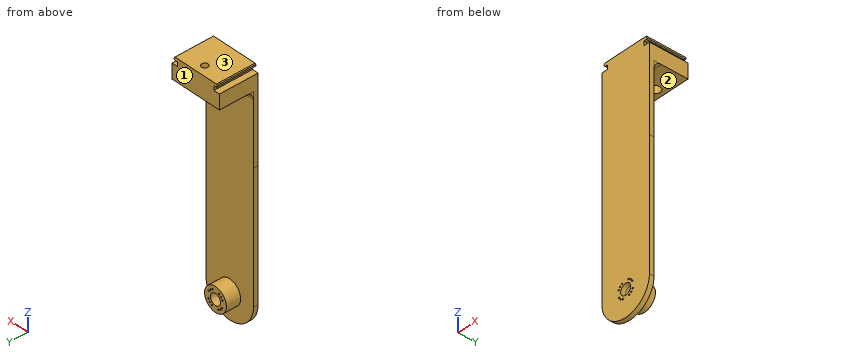
Autodesk Inventor part; units mm, degrees
ref_plane "YZ Plane" through (0, 0, 0) normal (1, 0, 0) x (0, 1, 0)
ref_plane "XZ Plane" through (0, 0, 0) normal (0, 1, 0) x (-1, 0, 0)
ref_plane "XY Plane" through (0, 0, 0) normal (0, 0, 1) x (1, 0, 0)
sketch "Sketch1" plane through (0, 0, 0) normal (0, 1, 0) x (-1, 0, 0)
  circle A0 centre (14, -52) radius 5.5 construction
  circle A1 centre (-14, -52) radius 5.5 construction
  circle A2 centre (-4.2824, 7.9159) radius 0.75 construction
  circle A3 centre (3.4651, 8.3062) radius 0.75 construction
  circle A4 centre (6.0357, 6.6761) radius 0.75 construction
  circle A5 centre (7.9159, 4.2824) radius 0.75 construction
  circle A6 centre (8.3062, -3.4651) radius 0.75 construction
  circle A7 centre (6.6761, -6.0357) radius 0.75 construction
  circle A8 centre (4.2824, -7.9159) radius 0.75 construction
  circle A9 centre (-3.4651, -8.3062) radius 0.75 construction
  circle A10 centre (-6.0357, -6.6761) radius 0.75 construction
  circle A11 centre (-7.9159, -4.2824) radius 0.75 construction
  circle A12 centre (-6.6761, 6.0357) radius 0.75 construction
  circle A13 centre (-8.3062, 3.4651) radius 0.75 construction
  circle A14 centre (0, 0) radius 6 construction
  line L0 (28, -68) -> (28, 0) construction
  arc A15 (28, 0) -> (-28, 0) centre (0, 0) ccw construction
  line L1 (-28, 0) -> (-28, -68) construction
  line L2 (-28, -68) -> (-22, -68) construction
  line L3 (-22, -68) -> (-22, -64) construction
  line L4 (-22, -64) -> (-24.8396, -64) construction
  line L5 (-24.8396, -64) -> (-25.8396, -63) construction
  line L6 (-25.8396, -63) -> (-25.8396, -61) construction
  line L7 (-25.8396, -61) -> (-24.8396, -60) construction
  line L8 (-24.8396, -60) -> (24.8396, -60) construction
  line L9 (24.8396, -60) -> (25.8396, -61) construction
  line L10 (25.8396, -61) -> (25.8396, -63) construction
  line L11 (25.8396, -63) -> (24.8396, -64) construction
  line L12 (24.8396, -64) -> (22, -64) construction
  line L13 (22, -64) -> (22, -68) construction
  line L14 (22, -68) -> (28, -68) construction
  line L15 (0, 0) -> (0, -300) construction
  line L16 (-28.3, 0) -> (-28.3, -300) construction
  line L17 (28.3, -300) -> (28.3, 0) construction
  arc A16 (28.3, 0) -> (-28.3, 0) centre (0, 0) ccw construction
  arc A17 (-28.3, -300) -> (28.3, -300) centre (0, -300) ccw construction
  line L18 (21.7, -63.7) -> (24.7153, -63.7)
  line L19 (24.7153, -63.7) -> (25.5396, -62.8757)
  line L20 (25.5396, -62.8757) -> (25.5396, -61.1243)
  line L21 (25.5396, -61.1243) -> (24.7153, -60.3)
  line L22 (24.7153, -60.3) -> (-24.7153, -60.3)
  line L23 (-24.7153, -60.3) -> (-25.5396, -61.1243)
  line L24 (-25.5396, -61.1243) -> (-25.5396, -62.8757)
  line L25 (-25.5396, -62.8757) -> (-24.7153, -63.7)
  line L26 (-24.7153, -63.7) -> (-21.7, -63.7)
  line L27 (-21.7, -63.7) -> (-21.7, -68.3)
  line L28 (-21.7, -68.3) -> (-28.3, -68.3) construction
  line L29 (-28.3, -68.3) -> (-28.3, 0) construction
  arc A18 (28.3, 0) -> (-28.3, 0) centre (0, 0) ccw construction
  line L30 (28.3, 0) -> (28.3, -68.3) construction
  line L31 (28.3, -68.3) -> (21.7, -68.3) construction
  line L32 (21.7, -68.3) -> (21.7, -63.7)
  arc A19 (-28.3, -300) -> (28.3, -300) centre (0, -300) ccw
  line L33 (0, -150) -> (28.3, -150) construction
  circle A20 centre (-4.2824, -307.9159) radius 0.75
  circle A21 centre (3.4651, -308.3062) radius 0.75
  circle A22 centre (6.0357, -306.6761) radius 0.75
  circle A23 centre (7.9159, -304.2824) radius 0.75
  circle A24 centre (8.3062, -296.5349) radius 0.75
  circle A25 centre (6.6761, -293.9643) radius 0.75
  circle A26 centre (4.2824, -292.0841) radius 0.75
  circle A27 centre (-3.4651, -291.6938) radius 0.75
  circle A28 centre (-6.0357, -293.3239) radius 0.75
  circle A29 centre (-7.9159, -295.7176) radius 0.75
  circle A30 centre (-6.6761, -306.0357) radius 0.75
  circle A31 centre (-8.3062, -303.4651) radius 0.75
  circle A32 centre (0, -300) radius 6
  line L34 (-28.3, -300) -> (-28.3, -68.3)
  line L35 (-28.3, -68.3) -> (-21.7, -68.3)
  line L36 (21.7, -68.3) -> (28.3, -68.3)
  line L37 (28.3, -68.3) -> (28.3, -300)
  point P0 (0, -150)
  dimension "d1" = 0.3
extrude "Extrusion1" add sketch "Sketch1" against normal blind 5
sketch "Sketch2" plane through (0, 0, 0) normal (0, 1, 0) x (1, 0, 0)
  circle A0 centre (0, 300) radius 6 construction
  circle A1 centre (8.3062, 303.4651) radius 0.75 construction
  circle A2 centre (6.6761, 306.0357) radius 0.75 construction
  circle A3 centre (-7.9159, 304.2824) radius 0.75 construction
  circle A4 centre (-6.0357, 306.6761) radius 0.75 construction
  circle A5 centre (-3.4651, 308.3062) radius 0.75 construction
  circle A6 centre (4.2824, 307.9159) radius 0.75 construction
  circle A7 centre (3.4651, 291.6938) radius 0.75 construction
  circle A8 centre (6.0357, 293.3239) radius 0.75 construction
  circle A9 centre (7.9159, 295.7176) radius 0.75 construction
  circle A10 centre (-8.3062, 296.5349) radius 0.75 construction
  circle A11 centre (-6.6761, 293.9643) radius 0.75 construction
  circle A12 centre (-4.2824, 292.0841) radius 0.75 construction
  arc A13 (28.3, 300) -> (-28.3, 300) centre (0, 300) ccw construction
  line L0 (-28.3, 300) -> (-28.3, 68.3) construction
  line L1 (-28.3, 68.3) -> (-21.7, 68.3)
  line L2 (-21.7, 68.3) -> (-21.7, 63.7)
  line L3 (-21.7, 63.7) -> (-24.7153, 63.7)
  line L4 (-24.7153, 63.7) -> (-25.5396, 62.8757)
  line L5 (-25.5396, 62.8757) -> (-25.5396, 61.1243)
  line L6 (-25.5396, 61.1243) -> (-24.7153, 60.3)
  line L7 (-24.7153, 60.3) -> (24.7153, 60.3)
  line L8 (24.7153, 60.3) -> (25.5396, 61.1243)
  line L9 (25.5396, 61.1243) -> (25.5396, 62.8757)
  line L10 (25.5396, 62.8757) -> (24.7153, 63.7)
  line L11 (24.7153, 63.7) -> (21.7, 63.7)
  line L12 (21.7, 63.7) -> (21.7, 68.3)
  line L13 (21.7, 68.3) -> (28.3, 68.3)
  line L14 (28.3, 68.3) -> (28.3, 300) construction
  line L15 (-28.3, 68.3) -> (-28.3, 300) construction
  line L16 (-28.3, 68.3) -> (-28.3, 84.3)
  line L17 (-28.3, 84.3) -> (28.3, 84.3)
  line L18 (28.3, 68.3) -> (28.3, 300) construction
  line L19 (28.3, 84.3) -> (28.3, 68.3)
  point P0 (0, 0)
  dimension "d5" = 16
extrude "Extrusion2" add sketch "Sketch2" along normal blind 37
sketch "Sketch3" plane through (0, 0, 0) normal (0, 1, 0) x (1, 0, 0)
  point P0 (0, 0)
sketch "Sketch4" plane through (0, 0, 0) normal (0, 1, 0) x (1, 0, 0)
  line L0 (-28.3, 84.3) -> (28.3, 84.3)
  line L1 (28.3, 84.3) -> (28.3, 300)
  arc A0 (28.3, 300) -> (-28.3, 300) centre (0, 300) ccw
  line L2 (-28.3, 300) -> (-28.3, 84.3)
  circle A1 centre (0, 300) radius 6
  circle A2 centre (8.3062, 303.4651) radius 0.75
  circle A3 centre (6.6761, 306.0357) radius 0.75
  circle A4 centre (-7.9159, 304.2824) radius 0.75
  circle A5 centre (-6.0357, 306.6761) radius 0.75
  circle A6 centre (-3.4651, 308.3062) radius 0.75
  circle A7 centre (4.2824, 307.9159) radius 0.75
  circle A8 centre (3.4651, 291.6938) radius 0.75
  circle A9 centre (6.0357, 293.3239) radius 0.75
  circle A10 centre (7.9159, 295.7176) radius 0.75
  circle A11 centre (-8.3062, 296.5349) radius 0.75
  circle A12 centre (-6.6761, 293.9643) radius 0.75
  circle A13 centre (-4.2824, 292.0841) radius 0.75
  circle A14 centre (0, 300) radius 13
  point P0 (0, 0)
  dimension "d8" = 26
extrude "Extrusion3" add sketch "Sketch4" along normal blind 15.5 contours A14
sketch "Sketch5" plane through (28.3, 0, -84.3) normal (0, 0, -1) x (-1, 0, 0)
  line L0 (56.6, 0) -> (0, 0) construction
  line L1 (56.6, 0) -> (56.6, 37) construction
  line L2 (0, 37) -> (56.6, 37) construction
  line L3 (0, 0) -> (0, 37) construction
  line L4 (0, 37) -> (56.6, 37) construction
  line L5 (28.3, 37) -> (28.3, 0) construction
  point P0 (28.3, 27)
  dimension "d11" = 10
hole "Hole1" at (0, 27, -84.3) direction (0, 0, 1) diameter 7 end through all counterbore diameter 11 counterbore depth 8
fillet "Fillet1" radius 8 1 edges at (0, 0, -84.3)
properties part number "arm_segment_1_2a"
Can you work these out from the model? Positions are in its coordinate system, mm. Face numbers are marked on the shaded views. Round coordinates to 2 decimals unless told otherwise and drop trailing zeros. Write each loop counter-clockwise with the first axis right and the second up, starting at its lowest first coordinate (ties: lowest second). Pieces come first, ordered by that corner, then holes. Notation, with made-up numbers: M -4.5,42 L 37.5,42 A37 ccw 37.5,81 Z; hole C 77.25,79.25 d1. An arc over 180 degrees is marked long. Use CSV: the item, a comma, the result in double quotes.
(1) I'm going to push flat-ended pins straight in: pin 1 (6 mm diameter, centred on x = 17, y = 16.5, fed in from -Z); pin 2 (3.5 mm diameter, centred on x = -26.5, y = 15.5, fed in from +Z); pin 3 (1.7 mm diameter, centred on x = 3.47, z = -291.69, fed in from +Y). Where does each tip first touch, or does it pass through?
Check values:
pin 1,"z = -84.3"
pin 2,"z = -60.33"
pin 3,"y = 15.5"
(2) Imagine slicing it at C-C (z = -215.5). Write out the boundary of the cut face in (x, y), plus the area to 3 significant figures.
Check values:
outline,"M -28.3,-5 L 28.3,-5 L 28.3,0 L -28.3,0 Z"
area,"283 mm^2"
(3) We'd pull the mould along Z, two halves only. Please class the marked faces 1, 2 and 3: +Z half, -Z half, draft (parallel to the pull), parting line (faces both ways), or undercut.
Check values:
face 1,"draft"
face 2,"undercut"
face 3,"+Z half"
(4) I need wall thicknesses on line 1 along Z through (x, y) = (0, 12.25); line 2 along Z through (x, y) = (-9.5, 19.5); line 3 along Y through (x, z) = (-8, -280.5). Which ranges of each line are inside material? Lowest first, please.
Check values:
line 1,"-313 to -306, -294 to -287, -84.3 to -60.3"
line 2,"-84.3 to -60.3"
line 3,"-5 to 0"
(5) Imagine slicing it at D-D (x = -17). Write out the boundary of the cut face in (y, z).
Check values:
outline,"M -5,-322.62 L 0,-322.62 L 0,-92.3 A8 cw 8,-84.3 L 37,-84.3 L 37,-60.3 L -5,-60.3 Z"
(6) Imagine slicing it at B-B (y = 27). Write out the boundary of the cut face in (x, z), plus the area to 3 significant figures.
Check values:
outline,"M -28.3,-84.3 L -5.5,-84.3 L -5.5,-76.3 L -3.5,-76.3 L -3.5,-60.3 L -24.72,-60.3 L -25.54,-61.12 L -25.54,-62.88 L -24.72,-63.7 L -21.7,-63.7 L -21.7,-68.3 L -28.3,-68.3 Z; M 3.5,-76.3 L 5.5,-76.3 L 5.5,-84.3 L 28.3,-84.3 L 28.3,-68.3 L 21.7,-68.3 L 21.7,-63.7 L 24.72,-63.7 L 25.54,-62.88 L 25.54,-61.12 L 24.72,-60.3 L 3.5,-60.3 Z"
area,"1,080 mm^2"
(7) Imagine slicing it at A-A (y = 5). Count the separate pieces of the cut face and the enclosed holes in it, plus the area to 3 significant figures.
Check values:
separate pieces,"2"
enclosed holes,"13"
area,"1,710 mm^2"
